The listing builds one solid part. Answer for the finished solid, in the listing's coordinates (mm). Face numbers are marked on the shaded views. A direction names the side the tool comes from. Round coordinates to 2 decimals unless told otherwise and drop trailing zeros. Write each loop counter-clockwise with the first axis right and the second up, starting at its lowest first coordinate (ties: lowest second). Pieces come first, ordered by that corner, then holes.
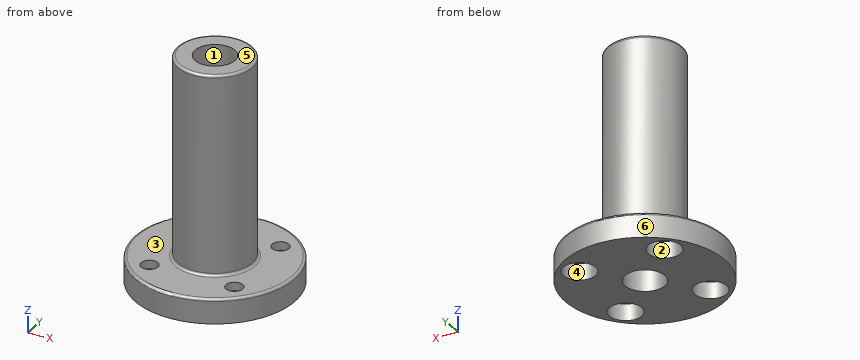
Autodesk Inventor part; units mm, degrees
ref_plane "YZ Plane" through (0, 0, 0) normal (1, 0, 0) x (0, 1, 0)
ref_plane "XZ Plane" through (0, 0, 0) normal (0, 1, 0) x (-1, 0, 0)
ref_plane "XY Plane" through (0, 0, 0) normal (0, 0, 1) x (1, 0, 0)
sketch "Sketch1" plane through (0, 0, 0) normal (0, 1, 0) x (-1, 0, 0)
  line L0 (0, 22.5) -> (7.5, 22.5)
  line L1 (7.5, 22.5) -> (7.5, -17.5)
  line L2 (7.5, -17.5) -> (16, -17.5)
  line L3 (16, -17.5) -> (16, -22.5)
  line L4 (16, -22.5) -> (0, -22.5)
  line L5 (0, -22.5) -> (0, 22.5)
  point P0 (0, 0)
  point P1 (0, 0)
  dimension "d0" = 7.5
  dimension "d1" = 5
  dimension "d3" = 16
  dimension "d4" = 45
revolve "Revolution1" add sketch "Sketch1" angle 360 about axis through (0, 0, -22.5) along (0, 0, 1)
sketch "Sketch2" plane through (0, 0, 22.5) normal (0, 0, 1) x (1, 0, 0)
  circle A0 centre (0, 0) radius 4
  dimension "d5" = 8
extrude "Extrusion1" cut sketch "Sketch2" against normal up to next
sketch "Sketch3" plane through (0, 0, -17.5) normal (0, 0, 1) x (1, 0, 0)
  circle A0 centre (-8.4853, 8.4853) radius 1.7
  line L0 (0, 0) -> (-8.4853, 8.4853) construction
  line L1 (0, 0) -> (-3.1591, 0)
  circle A1 centre (-8.4853, -8.4853) radius 1.7
  circle A2 centre (8.4853, -8.4853) radius 1.7
  circle A3 centre (8.4853, 8.4853) radius 1.7
  dimension "d8" = 3.4
  dimension "d9" = 12
  dimension "d10" = 45
  dimension "d13" = 360
extrude "Extrusion2" cut sketch "Sketch3" against normal up to next
sketch "Sketch4" plane through (0, 0, -22.5) normal (0, 0, -1) x (-1, 0, 0)
  circle A0 centre (8.4853, 8.4853) radius 1.7
  circle A1 centre (8.4853, 8.4853) radius 3.25
  circle A2 centre (-8.4853, 8.4853) radius 3.25
  circle A3 centre (-8.4853, -8.4853) radius 3.25
  circle A4 centre (8.4853, -8.4853) radius 3.25
  point P0 (0, 0)
  dimension "d17" = 6.5
  dimension "d20" = 360
extrude "Extrusion3" cut sketch "Sketch4" against normal blind 3.3
fillet "Fillet1" radius 0.5 3 edges at (7.5, 0, -17.5) (16, 0, -17.5) (7.5, 0, 22.5)
properties part number "LMF8LUU"
1. Section C-C on z = 17 is taken. Determine the outline of the cut face in (x, y).
Geometry says:
outline: circle Ø15 at (0, 0); hole circle Ø8 at (0, 0)
2. A tool of negligible diameter and unlimited length cuts with its end or side. For the marked faces 1, 2 and 3, from which of +Z, -Z, +X, -X, +Y, -Y can it reach the whole face along a straight path? Write none if from no direction.
Geometry says:
face 1: +Z, -Z
face 2: -Z
face 3: +Z
3. Given pin 1 (2 mm diameter, centred on x = 9.5, y = -9.5, fed in from -Z); pin 2 (5 mm diameter, centred on x = -12, y = 1.5, fed in from +Z); pin 3 (3 mm diameter, centred on x = 8.49, y = -8.49, fed in from -Z); pin 4 (5 mm diameter, centred on x = -4.5, z = -1, fed in from -Y), each flat-ended and moving along its own axis, determine where each tip first touches the part or whether it passes through.
Geometry says:
pin 1: stops at z = -19.2
pin 2: stops at z = -17.5
pin 3: passes through
pin 4: stops at y = -7.23
4. Section A-A on y = 0 is taken. Determine the outline of the cut face in (x, z).
Geometry says:
outline: (-16, -22.5) - (-4, -22.5) - (-4, 22.5) - (-7, 22.5) arc R0.5 ccw to (-7.5, 22) - (-7.5, -17) arc R0.5 cw to (-8, -17.5) - (-15.5, -17.5) arc R0.5 ccw to (-16, -18) - close; (4, -22.5) - (16, -22.5) - (16, -18) arc R0.5 ccw to (15.5, -17.5) - (8, -17.5) arc R0.5 cw to (7.5, -17) - (7.5, 22) arc R0.5 ccw to (7, 22.5) - (4, 22.5) - close
5. For a pull along Y with two mould halves and no side action, classify the marked faces 4, 5 and 6 as released by +Y, released by -Y, zero draft, split by the parting line, or undercut.
Geometry says:
face 4: undercut
face 5: zero draft
face 6: split by the parting line
6. Straight lines are drawn through the part: line 1 along Z through (x, y) = (2, 10); line 2 along X through (y, z) = (2.5, 20.5); line 3 along Y through (x, z) = (-3, 9.5). For each, find the intervals that lie inside material, in ascending order.
Geometry says:
line 1: z = -22.5 to -17.5
line 2: x = -7.07 to -3.12, 3.12 to 7.07
line 3: y = -6.87 to -2.65, 2.65 to 6.87
